from build123d import *

# Parameters (mm, degrees)
BOSS_EXTRUDE1_DEPTH = 6.35
SKETCH2_W           = 4.7625
SKETCH2_H           = 19.05
CUT_EXTRUDE1_DEPTH  = 4.7625
FILLET1_R           = 1.27


with BuildPart() as part:
    # Sketch1 → Boss-Extrude1 (new body)
    with BuildSketch(Plane(origin=(0, 0, 0), x_dir=(1, 0, 0), z_dir=(0, 1, 0))):
        with BuildLine():
            Line((11.90625, 25.4), (16.51, 25.4))
            ThreePointArc((16.51, 25.4), (18.306051224, 24.656051224), (19.05, 22.86))
            Line((19.05, 22.86), (19.05, 2.54))
            ThreePointArc((19.05, 2.54), (18.306051224, 0.743948776), (16.51, 0))
            Line((16.51, 0), (2.54, 0))
            ThreePointArc((2.54, 0), (0.743948776, 0.743948776), (0, 2.54))
            Line((0, 2.54), (0, 22.86))
            ThreePointArc((0, 22.86), (0.743948776, 24.656051224), (2.54, 25.4))
            Line((2.54, 25.4), (7.14375, 25.4))
            Line((7.14375, 25.4), (7.14375, 19.05))
            Line((7.14375, 19.05), (11.90625, 19.05))
            Line((11.90625, 19.05), (11.90625, 25.4))
        make_face()
    extrude(amount=BOSS_EXTRUDE1_DEPTH)

    # Sketch2 → Cut-Extrude1 (cut)
    with BuildSketch(Plane(origin=(0, 6.35, 0), x_dir=(1, 0, 0), z_dir=(0, 1, 0))):
        with Locations((9.525, 9.525)):
            Rectangle(SKETCH2_W, SKETCH2_H)
    extrude(amount=-CUT_EXTRUDE1_DEPTH, mode=Mode.SUBTRACT)

    # Fillet1
    fillet1_edges = [part.edges().sort_by_distance(p)[0] for p in [
        (0.743948776, 6.35, -24.656051224),
        (4.841875, 6.35, -25.4),
        (14.208125, 6.35, -25.4),
        (14.208125, 6.35, 0),
        (18.306051224, 6.35, -24.656051224),
        (7.14375, 3.96875, 0),
        (9.525, 1.5875, -19.05),
        (9.525, 1.5875, 0),
        (11.90625, 3.96875, 0),
        (19.05, 6.35, -12.7),
        (18.306051224, 6.35, -0.743948776),
        (4.841875, 6.35, 0),
        (0.743948776, 6.35, -0.743948776),
        (0, 6.35, -12.7),
    ]]
    fillet(fillet1_edges, radius=FILLET1_R)


solid = part.part
Geometry: final body of the model. Coordinates: model frame, mm. A direction names the side the tool comes from. Round coordinates to 2 decimals unless told otherwise and drop trailing zeros. Order: outer loops, then holes, each group sorted by start corner. A loop starts at its lowest first (then second) coordinate and runs counter-clockwise, first axis right, second up.
Q1. Section B-B, the plane x = 8.75. Output: boundary loops of the cut face in (y, z).
Result sheet:
outline: (0, -19.05) - (0.32, -19.05) arc R1.27 ccw to (1.59, -17.78) - (1.59, -1.27) arc R1.27 ccw to (0.32, 0) - (0, 0) - close
Q2. Mould query, pull axis X, two halves, no side actions, for faces 3 (the face through (19.05, 3, -13)), 4 (the face through (10, 0, -13)), 5 (the face through (9, 1.587, -10)). Classes: released by +X, released by -X, zero draft, split by the parting line, or undercut.
Result sheet:
face 3: released by +X
face 4: zero draft
face 5: undercut
Q3. Pin query (flat end, axial travel): pin 1 (2.5 mm diameter, centred on x = 8.5, z = -12.5, fed in from +Y); pin 2 (2 mm diameter, centred on x = 15.5, z = -22, fed in from -Y). Return the tip coordinate at first contact, or that it passes through.
Result sheet:
pin 1: stops at y = 1.59
pin 2: stops at y = 0
Q4. Section A-A, the plane z = -21.75. Output: boundary loops of the cut face in (x, y), and give its area (3 significant figures).
Result sheet:
outline: (0, 0) - (7.14, 0) - (7.14, 6.35) - (1.27, 6.35) arc R1.27 ccw to (0, 5.08) - close; (11.91, 0) - (19.05, 0) - (19.05, 5.08) arc R1.27 ccw to (17.78, 6.35) - (11.91, 6.35) - close
area: 90.0 mm2
Q5. Material intervals for probe 1 along X at (y, z) = (1, -21); probe 2 along X at (y, z) = (6, -13.25); probe 3 along Y at (x, z) = (8, -14.25), sorted ascending.
Result sheet:
probe 1: x = 0 to 7.14, 11.91 to 19.05
probe 2: x = 0.39 to 7.14, 11.91 to 18.66
probe 3: y = 0 to 1.59
Q6. Section C-C, the plane y = 0.75. Output: boundary loops of the cut face in (x, z).
Result sheet:
outline: (0, -22.86) arc R2.54 ccw to (2.54, -25.4) - (7.14, -25.4) - (7.14, -18.97) - (11.91, -18.97) - (11.91, -25.4) - (16.51, -25.4) arc R2.54 ccw to (19.05, -22.86) - (19.05, -2.54) arc R2.54 ccw to (16.51, 0) - (13.18, 0) arc R1.27 ccw to (12.74, -0.08) - (6.31, -0.08) arc R1.27 ccw to (5.87, 0) - (2.54, 0) arc R2.54 ccw to (0, -2.54) - close
Q7. Section D-D, the plane z = -17.5. Output: boundary loops of the cut face in (x, y).
Result sheet:
outline: (0, 0) - (19.05, 0) - (19.05, 5.08) arc R1.27 ccw to (17.78, 6.35) - (11.91, 6.35) - (11.91, 1.59) - (7.14, 1.59) - (7.14, 6.35) - (1.27, 6.35) arc R1.27 ccw to (0, 5.08) - close
Q8. Access query for faces 1 (the face through (9.576, 1.206, -0.362)), 2 (the face through (15, 6.35, -13)). Directions: +Z, -Z, +X, -X, +Y, -Y. A direction counts if a zero-diameter tool reaches every point of the face in a straight line with its end or side. Return the directions, or none.
Result sheet:
face 1: +Z, +Y
face 2: +Z, -Z, +X, -X, +Y
